Here's the drawing with two shaded views (mm, measured from the low corner). I have some questions. A direction names the side the tool comes from. Give positions to 0.01 mm unless a question says otherwise; leave off trailing zeros. Loops run counter-clockwise (first coordinate to the right, second up) from the corner with the lowest first, then second, coordinate; pieces in that order, holes last. Notation, with made-up numbers: M 69,-15 L 119,-15 A24 cw 119,5 Z; hole C -6,21.5 d11. An arc over 180 degrees is marked long. Use a Markdown table: item, result. Add a question column.
1) If I drill on line 1 along Y through (x, z) = (246, 227.5); line 2 along Z through (x, y) = (174.5, 156.5); line 3 along Z through (x, y) = (119.5, 178), over which ranges is the centre line in solid material (lowest first)? Write a range as [from, to].
2) Will these pins go through, and if not, where does the flat tip stop? pin 1 Ø8 at (y, z) = (483, 80) entering from -X; pin 2 Ø3 at (y, z) = (276.5, 275.5) entering from +X; pin 3 Ø4 at (y, z) = (523.5, 55) entering from +X.
3) Suppose I cut it at D-D on y = 217.5. List the corners of the cut face in (x, z) for me, and give its area (3 significant figures).
4) Suppose I cut it at B-B on z = 135. List the corners of the cut face in (x, y) for me.
5) Which directions (+Z, -Z, +X, -X, +Y, -Y) give clear straight access to the entire face, cutting with the end or side of a thin tool? Please do the marked faces 1, 2, 3, 4 and 5.
6) Suppose I cut it at C-C on x = 175. List the corners of the cut face in (y, z) for me, and give its area (3 significant figures).
7) Suppose I cut it at A-A on y = 300. List the corners of the cut face in (x, z) for me.
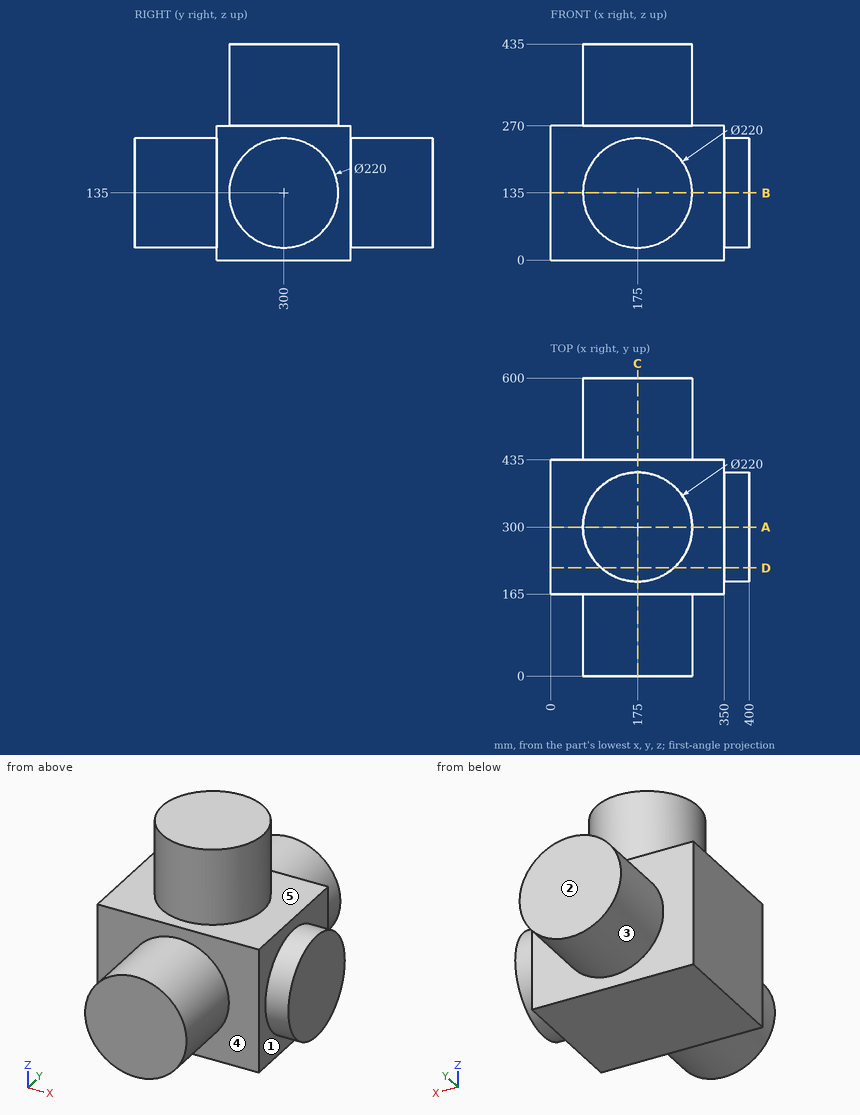
Answer block:
| question | item | result |
|---|---|---|
| 1 | line 1 | y = [165, 435] |
| 1 | line 2 | z = [25, 245] |
| 1 | line 3 | z = [0, 270] |
| 2 | pin 1 | stops at x = 77.54 |
| 2 | pin 2 | stops at x = 282.78 |
| 2 | pin 3 | stops at x = 252.56 |
| 3 | outline | M 0,0 L 350,0 L 350,62.24 L 400,62.24 L 400,207.76 L 350,207.76 L 350,270 L 247.76,270 L 247.76,435 L 102.24,435 L 102.24,270 L 0,270 Z |
| 3 | area | 126,000 mm^2 |
| 4 | outline | M 0,165 L 65,165 L 65,0 L 285,0 L 285,165 L 350,165 L 350,190 L 400,190 L 400,410 L 350,410 L 350,435 L 285,435 L 285,600 L 65,600 L 65,435 L 0,435 Z |
| 5 | face 1 | +X |
| 5 | face 2 | +Z, -Z, +X, -X, +Y |
| 5 | face 3 | +Y |
| 5 | face 4 | -Y |
| 5 | face 5 | +Z |
| 6 | outline | M 0,25 L 165,25 L 165,0 L 435,0 L 435,25 L 600,25 L 600,245 L 435,245 L 435,270 L 410,270 L 410,435 L 190,435 L 190,270 L 165,270 L 165,245 L 0,245 Z |
| 6 | area | 182,000 mm^2 |
| 7 | outline | M 0,0 L 350,0 L 350,25 L 400,25 L 400,245 L 350,245 L 350,270 L 285,270 L 285,435 L 65,435 L 65,270 L 0,270 Z |
